from build123d import *

# Parameters (mm, degrees)
SKETCH2_W                                  = 220
SKETCH2_H                                  = 220
BOSS_EXTRUDE1_DEPTH                        = 15.875
SKETCH4_W                                  = 108
SKETCH4_H                                  = 108
CUT_EXTRUDE1_DEPTH                         = 7.9375
FILLET1_R                                  = 12.5
SKETCH5_R                                  = 5.55625
CUT_EXTRUDE2_DEPTH                         = 156.765862455
MIRROR1_AT_THE_SECOND_PLANE_COPY_1_SKETC_R = 5.55625
MIRROR1_AT_THE_SECOND_PLANE_COPY_1_DEPTH   = 156.765862455
SKETCH6_R                                  = 16.51
CUT_EXTRUDE3_DEPTH                         = 156.765862455


with BuildPart() as part:
    # Sketch2 → Boss-Extrude1 (new body)
    with BuildSketch(Plane.XY):
        Rectangle(SKETCH2_W, SKETCH2_H)
    extrude(amount=BOSS_EXTRUDE1_DEPTH)

    # Sketch4 → Cut-Extrude1 (cut)
    with BuildSketch(Plane.XY.offset(15.875)):
        Rectangle(SKETCH4_W, SKETCH4_H)
    extrude(amount=-CUT_EXTRUDE1_DEPTH, mode=Mode.SUBTRACT)

    # Fillet1
    fillet1_edges = [part.edges().sort_by_distance(p)[0] for p in [
        (-54, -54, 11.90625),
        (-54, 54, 11.90625),
        (54, 54, 11.90625),
        (54, -54, 11.90625),
    ]]
    fillet(fillet1_edges, radius=FILLET1_R)

    # Sketch5 → Cut-Extrude2 (cut, through all)
    with BuildSketch(Plane.XY.offset(7.9375)):
        with Locations((-41.5, 41.5)):
            Circle(SKETCH5_R)
    cut_extrude2 = extrude(amount=-CUT_EXTRUDE2_DEPTH, mode=Mode.SUBTRACT)

    # Mirror1: Cut-Extrude2 across plane
    add(cut_extrude2.mirror(Plane.ZX), mode=Mode.SUBTRACT)

    # Mirror1 at the second plane: Cut-Extrude2 across plane
    add(cut_extrude2.mirror(Plane(origin=(0, 0, 0), x_dir=(0, 0, 1), z_dir=(1, 0, 0))), mode=Mode.SUBTRACT)

    # Mirror1 at the second plane copy 1 sketc → Mirror1 at the second plane copy 1 (cut, through all)
    with BuildSketch(Plane(origin=(0, 0, 7.9375), x_dir=(-1, 0, 0), z_dir=(0, 0, 1))):
        with Locations((-41.5, 41.5)):
            Circle(MIRROR1_AT_THE_SECOND_PLANE_COPY_1_SKETC_R)
    extrude(amount=-MIRROR1_AT_THE_SECOND_PLANE_COPY_1_DEPTH, mode=Mode.SUBTRACT)

    # Sketch6 → Cut-Extrude3 (cut, through all)
    with BuildSketch(Plane.XY.offset(7.9375)):
        Circle(SKETCH6_R)
    extrude(amount=-CUT_EXTRUDE3_DEPTH, mode=Mode.SUBTRACT)


solid = part.part
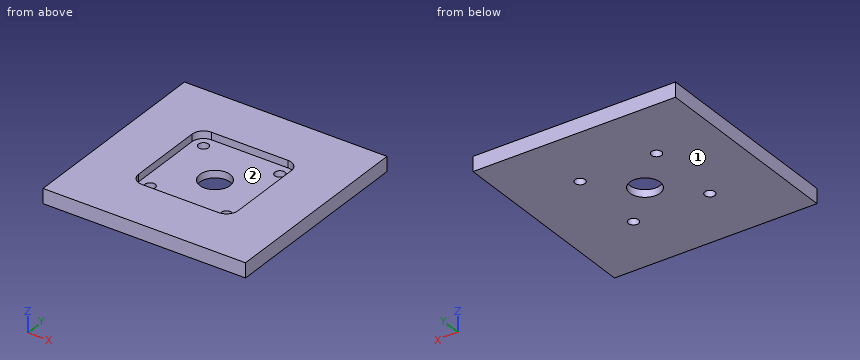
Can you work these out from the model? Positions are in its coordinate system, mm. Face numbers are marked on the shaded views. Give positions to 0.01 mm unless a question says otherwise; leave off trailing zeros. Loops run counter-clockwise (first coordinate to the right, second up) from the corner with the lowest first, then second, coordinate; pieces in that order, holes last. Notation, with made-up numbers: (76.5, 27.5) -> (95.5, 27.5) arc R25 cw to (95.5, 61.5) -> close; hole circle Ø7 at (-7.5, 57). An arc over 180 degrees is marked (long way). Use one line per item in the form item = value.
1) Will this pin go through, and if not, where does the flat tip stop? pin 1 (14.5 mm diameter, centred on x = -41.5, y = 41.5, fed in from +Z).
Answers:
pin_1 = 7.94
2) I need wall thicknesses on line 1 along Y through (x, z) = (-41.5, 2); line 2 along Y through (x, z) = (0, 1.75); line 3 along Y through (x, z) = (0, 14). Which ranges of each line are inside material? Lowest first, please.
Answers:
line_1 = -110 to -47.06, -35.94 to 35.94, 47.06 to 110
line_2 = -110 to -16.51, 16.51 to 110
line_3 = -110 to -54, 54 to 110
3) We'd pull the mould along Y, two halves only. Please class the marked faces 1 and 2: released by +Y, released by -Y, zero draft, split by the parting line, or undercut.
Answers:
face_1 = zero draft
face_2 = undercut
4) If we section it at C-C (x = -44): Please give me the cut outline in (y, z) (1 decimal).
Answers:
outline = (-110, 0) -> (-46.5, 0) -> (-46.5, 7.9) -> (-53.7, 7.9) -> (-53.7, 15.9) -> (-110, 15.9) -> close; (-36.5, 0) -> (36.5, 0) -> (36.5, 7.9) -> (-36.5, 7.9) -> close; (46.5, 0) -> (110, 0) -> (110, 15.9) -> (53.7, 15.9) -> (53.7, 7.9) -> (46.5, 7.9) -> close
5) If we section it at B-B (z = 4): Please give me the cut outline in (x, y), plus the area to 3 significant figures.
Answers:
outline = (-110, -110) -> (110, -110) -> (110, 110) -> (-110, 110) -> close; hole circle Ø11.11 at (-41.5, -41.5); hole circle Ø11.11 at (-41.5, 41.5); hole circle Ø33.02 at (0, 0); hole circle Ø11.11 at (41.5, -41.5); hole circle Ø11.11 at (41.5, 41.5)
area = 47,200 mm²
6) If we section it at A-A (y = 0): Please give me the cut outline in (x, z) (1 decimal).
Answers:
outline = (-110, 0) -> (-16.5, 0) -> (-16.5, 7.9) -> (-54, 7.9) -> (-54, 15.9) -> (-110, 15.9) -> close; (16.5, 0) -> (110, 0) -> (110, 15.9) -> (54, 15.9) -> (54, 7.9) -> (16.5, 7.9) -> close
7) If we section it at D-D (y = 25): Please give me the cut outline in (x, z) (1 decimal).
Answers:
outline = (-110, 0) -> (110, 0) -> (110, 15.9) -> (54, 15.9) -> (54, 7.9) -> (-54, 7.9) -> (-54, 15.9) -> (-110, 15.9) -> close
